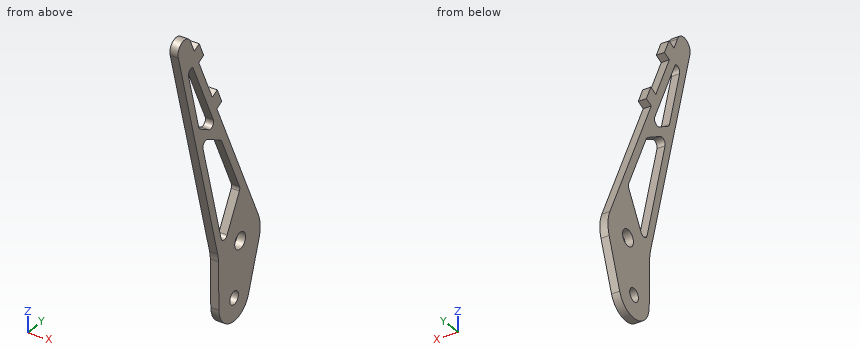
```python
from build123d import *

# Parameters (mm, degrees)
SKETCH1_R           = 4
SKETCH1_R_2         = 5
BOSS_EXTRUDE1_DEPTH = 5
FILLET3_R           = 20
FILLET10_R          = 3


with BuildPart() as part:
    # Sketch1 → Boss-Extrude1 (new body)
    # profile 1 of 3: a face of its own
    with BuildSketch(Plane.YZ):
        with BuildLine():
            Line((-14.443258315, 31.513848096), (-13.998623919, -0.196286448))
            ThreePointArc((-13.998623919, -0.196286448), (-2.196477435, -13.826622396), (13.248647006, -4.52474889))
            Line((13.248647006, -4.52474889), (25.556741685, 31.513848096))
            Line((25.556741685, 31.513848096), (-15.913444308, 121.828294459))
            Line((-15.913444308, 121.828294459), (-17.991906384, 126.354803013))
            Line((-17.991906384, 126.354803013), (-20.086315573, 130.916041451))
            Line((-20.086315573, 130.916041451), (-32.596955812, 158.161917487))
            Line((-32.596955812, 158.161917487), (-34.683391444, 162.705790984))
            Line((-34.683391444, 162.705790984), (-36.769827077, 167.24966448))
            Line((-36.769827077, 167.24966448), (-40.108124089, 174.519862074))
            ThreePointArc((-40.108124089, 174.519862074), (-47.798400673, 178.105896939), (-51.384435538, 170.415620354))
            Line((-51.384435538, 170.415620354), (-14.443258315, 31.513848096))
        make_face()
        with Locations(Location((0, 0, 0), (0, 0, 270))):
            Circle(SKETCH1_R, mode=Mode.SUBTRACT)
        with Locations(Location((5.556741685, 31.513848096, 0), (0, 0, 270))):
            Circle(SKETCH1_R_2, mode=Mode.SUBTRACT)
        Polygon((-10.059219018, 34.483430451), (-30.486505123, 111.291655193), (-11.718080145, 100.709404741), (5.599975549, 62.99386104), align=None, mode=Mode.SUBTRACT)
        Polygon((-38.215011053, 158.414852351), (-15.274502195, 108.454638594), (-32.282363467, 118.044225778), (-44.116299331, 162.540768328), align=None, mode=Mode.SUBTRACT)
    # profile 2 of 3: a face of its own
    with BuildSketch(Plane.YZ):
        Polygon((-17.991906384, 126.354803013), (-15.913444308, 121.828294459), (-11.369603993, 123.914714855), (-15.542475258, 133.002461848), (-20.086315573, 130.916041451), align=None)
    # profile 3 of 3: a face of its own
    with BuildSketch(Plane.YZ):
        Polygon((-32.22595358, 169.336100113), (-36.769827077, 167.24966448), (-34.683391444, 162.705790984), (-32.596955812, 158.161917487), (-28.053082315, 160.24835312), align=None)
    extrude(amount=-BOSS_EXTRUDE1_DEPTH)

    # Fillet3
    fillet3_edges = [part.edges().sort_by_distance(p)[0] for p in [
        (-2.5, 25.556741685, 31.513848096),
        (-2.5, -14.443258315, 31.513848096),
    ]]
    fillet(fillet3_edges, radius=FILLET3_R)

    # Fillet10
    # the kernel refuses this fillet: 3 mm, written as the material it adds along each edge
    with BuildSketch(Plane(origin=(0, -38.215011053, 158.414852351), x_dir=(0, 0.41728712651347166, -0.9087746992770703), z_dir=(-1, 0, 0))) as fillet10_piece_1:
        with BuildLine():
            CenterArc((FILLET10_R * 0.271478941521, FILLET10_R), FILLET10_R, 239.62294962, 30.37705038)
            Line((-FILLET10_R * 0.23420930525, FILLET10_R * 0.137283709973), (0, 0))
            Line((0, 0), (FILLET10_R * 0.271478941521, 0))
        make_face()
    extrude(amount=5)
    with BuildSketch(Plane(origin=(0, -32.282363467, 118.044225778), x_dir=(0, 0.8710790696902164, -0.49114280443433855), z_dir=(-1, 0, 0))) as fillet10_piece_2:
        with BuildLine():
            CenterArc((FILLET10_R * 0.421297147858, -FILLET10_R), FILLET10_R, 90, 45.691106369)
            Line((-FILLET10_R * 0.294287167004, -FILLET10_R * 0.301473630904), (0, 0))
            Line((0, 0), (FILLET10_R * 0.421297147858, 0))
        make_face()
    extrude(amount=5)
    with BuildSketch(Plane(origin=(0, -30.486505123, 111.291655193), x_dir=(0, 0.25701761253564515, -0.9664067191645953), z_dir=(-1, 0, 0))) as fillet10_piece_3:
        with BuildLine():
            CenterArc((FILLET10_R * 2.37362157585, -FILLET10_R), FILLET10_R, 90, 134.308893631)
            Line((FILLET10_R * 1.65803726099, -FILLET10_R * 1.6985263691), (0, 0))
            Line((0, 0), (FILLET10_R * 2.37362157585, 0))
        make_face()
    extrude(amount=5)
    with BuildSketch(Plane(origin=(0, -11.718080145, 100.709404741), x_dir=(0, -0.8710790696902125, 0.4911428044343457), z_dir=(-1, 0, 0))) as fillet10_piece_4:
        with BuildLine():
            CenterArc((FILLET10_R * 0.324156203472, -FILLET10_R), FILLET10_R, 90, 35.920846961)
            Line((-FILLET10_R * 0.262510846562, -FILLET10_R * 0.190171763641), (0, 0))
            Line((0, 0), (FILLET10_R * 0.324156203472, 0))
        make_face()
    extrude(amount=5)
    with BuildSketch(Plane(origin=(0, -10.059219018, 34.483430451), x_dir=(0, -0.2570176125356449, 0.9664067191645953), z_dir=(-1, 0, 0))) as fillet10_piece_5:
        with BuildLine():
            CenterArc((FILLET10_R * 2.49571060233, FILLET10_R), FILLET10_R, 133.670716463, 136.329283537)
            Line((FILLET10_R * 1.80519778573, FILLET10_R * 1.72332015741), (0, 0))
            Line((0, 0), (FILLET10_R * 2.49571060233, 0))
        make_face()
    extrude(amount=5)
    with BuildSketch(Plane(origin=(0, 5.599975549, 62.99386104), x_dir=(0, -0.41728712651347205, 0.9087746992770702), z_dir=(-1, 0, 0))) as fillet10_piece_6:
        with BuildLine():
            CenterArc((FILLET10_R * 0.503395718442, -FILLET10_R), FILLET10_R, 90, 53.440975871)
            Line((-FILLET10_R * 0.299847949894, -FILLET10_R * 0.404349423506), (0, 0))
            Line((0, 0), (FILLET10_R * 0.503395718442, 0))
        make_face()
    extrude(amount=5)
    with BuildSketch(Plane(origin=(0, -15.274502195, 108.454638594), x_dir=(0, -0.4172871265134709, 0.9087746992770708), z_dir=(-1, 0, 0))) as fillet10_piece_7:
        with BuildLine():
            CenterArc((FILLET10_R * 3.08493247789, -FILLET10_R), FILLET10_R, 90, 144.079153039)
            Line((FILLET10_R * 2.49826542786, -FILLET10_R * 1.80982823636), (0, 0))
            Line((0, 0), (FILLET10_R * 3.08493247789, 0))
        make_face()
    extrude(amount=5)
    with BuildSketch(Plane(origin=(0, -44.116299331, 162.540768328), x_dir=(0, 0.2570176125356455, -0.9664067191645951), z_dir=(-1, 0, 0))) as fillet10_piece_8:
        with BuildLine():
            CenterArc((FILLET10_R * 2.73652664972, -FILLET10_R), FILLET10_R, 90, 139.852690212)
            Line((FILLET10_R * 2.09177163516, -FILLET10_R * 1.76438927988), (0, 0))
            Line((0, 0), (FILLET10_R * 2.73652664972, 0))
        make_face()
    extrude(amount=5)


solid = part.part
```
Build history of the part. All positions in model axes, mm. Give positions to 0.01 mm unless a question says otherwise; leave off trailing zeros. Loops run counter-clockwise (first coordinate to the right, second up) from the corner with the lowest first, then second, coordinate; pieces in that order, holes last. Notation, with made-up numbers: (-27, -37) - (17, -37) arc R27 cw to (17, -21) - close; hole circle Ø4 at (78, 30). An arc over 180 degrees is marked (long way). Use a Markdown table: item, result.
(1) Drop flat-ended pins along their axis: pin 1 Ø6 at (y, z) = (5.56, 31.51) entering from +X; pin 2 Ø8 at (y, z) = (-15, 54.5) entering from -X; pin 3 Ø1 at (x, z) = (-3.5, 144.5) entering from +Y; pin 4 Ø2 at (x, z) = (-3.5, 127) entering from -Y. Give the stop position or say it passes through.
Taken from the geometry:
| item | result |
|---|---|
| pin 1 | through |
| pin 2 | x = -5 |
| pin 3 | y = -26.09 |
| pin 4 | y = -40.1 |
(2) Band-saw the part on C-C (z = 68.5). Give the cut face in (x, y).
Taken from the geometry:
| item | result |
|---|---|
| outline | (-5, -24.28) - (0, -24.28) - (0, -19.11) - (-5, -19.11) - close; (-5, 3.07) - (0, 3.07) - (0, 8.57) - (-5, 8.57) - close |
(3) Wall check: line 1 along Y through (x, z) = (-0.15, 56); line 2 along Y through (x, z) = (-1.3, 0); line 3 along Y through (x, z) = (-1.5, 9). Give the ranges that are in metal, low to high.
Taken from the geometry:
| item | result |
|---|---|
| line 1 | -20.96 to -15.78, 1.76 to 14.31 |
| line 2 | -14 to -4, 4 to 14.79 |
| line 3 | -14.13 to 17.87 |
(4) Band-saw the part on B-B (x = -2.7). Give the number of separate pieces and of enclosed holes in the cut face, and give its area (3 significant figures).
Taken from the geometry:
| item | result |
|---|---|
| separate pieces | 1 |
| enclosed holes | 4 |
| area | 3,610 mm2 |
(5) Band-saw the part on A-A (y = 7.5). Give the cut face in (x, z).
Taken from the geometry:
| item | result |
|---|---|
| outline | (-5, -11.82) - (0, -11.82) - (0, 26.91) - (-5, 26.91) - close; (-5, 36.12) - (0, 36.12) - (0, 70.84) - (-5, 70.84) - close |
(6) Band-saw the part on D-D (z = 14.5). Give the cut face in (x, y).
Taken from the geometry:
| item | result |
|---|---|
| outline | (-5, -14.2) - (0, -14.2) - (0, 19.75) - (-5, 19.75) - close |
